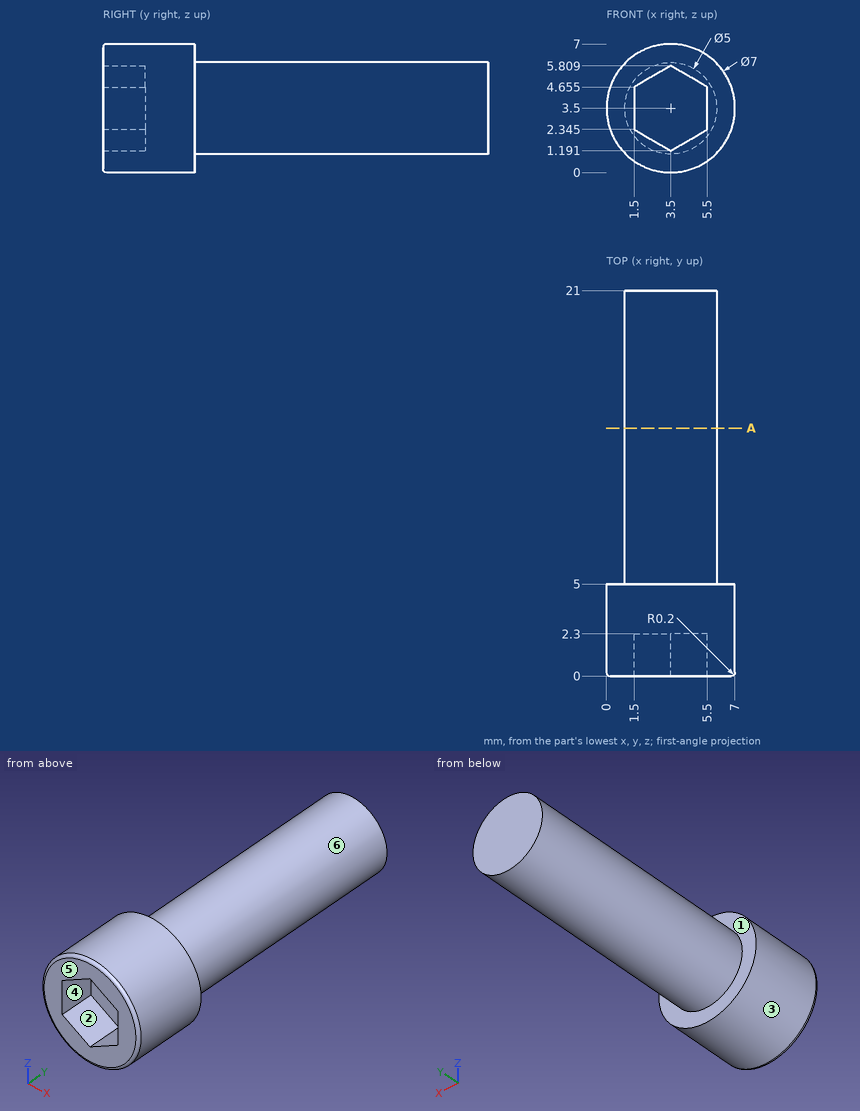
The figure shows three views and two pictorial views of one solid part (mm, origin at its lowest corner). Answer the questions. A direction names the side the tool comes from. Give positions to 0.01 mm unless a question says otherwise; leave off trailing zeros. Order: outer loops, then holes, each group sorted by start corner. A loop starts at its lowest first (then second) coordinate and runs counter-clockwise, first axis right, second up. Notation, with made-up numbers: (0, 32.5) -> (7, 32.5) arc R26 ccw to (7, 48.5) -> close; hole circle Ø5 at (12.25, 77). An arc over 180 degrees is marked (long way). Answer as CSV lines item,"result". Start each with the question number.
Q1. Find the intervals of material crossed by L1, parallel to Z at x = 2, y = 9; L2, parallel to Y at x = 4.5, z = 4.5, in increasing order.
Q2. Determine the mould class of the marked faces 4, 5 and 6 for opening direction X: pulls with the +X half, pulls with the -X half, needs draft (parallel to the pull), parting line crosses it, or undercut.
Q3. Given pin 1 (1.2 mm diameter, centred on x = 3, z = 3.5, fed in from -Y); pin 2 (1 mm diameter, centred on y = 9.5, z = 6, fed in from +X); pin 3 (1.5 mm diameter, centred on y = 12, z = 4.5, fed in from -X), each flat-ended and moving along its own axis, determine where each tip first touches the part or whether it passes through.
Q4. A cutting plane is placed at A-A (y = 13.5). Determine the outline of the cut face in (x, z).
Q5. Which of the six approach directions +Z, -Z, +X, -X, +Y, -Y give full straight-line access (tool end or side, diameter ignored) to the marked faces 1, 2 and 3?
Results found:
1,L1,"1.5 to 5.5"
1,L2,"2.3 to 21"
2,face 4,"undercut"
2,face 5,"needs draft"
2,face 6,"parting line crosses it"
3,pin 1,"y = 2.3"
3,pin 2,"x = 5"
3,pin 3,"x = 1.01"
4,outline,"circle Ø5 at (3.5, 3.5)"
5,face 1,"+Y"
5,face 2,"-Y"
5,face 3,"+Y, -Y"
